```python
from build123d import *

# Parameters (mm, degrees)
F0_R     = 1.671135
F1_DEPTH = 7


with BuildPart() as f1:
    # F0 (on Top) → F1 (new body)
    with BuildSketch(Plane.XY):
        with BuildLine():
            ThreePointArc((5.710763, 3.295388), (5.423242, 3.744527), (5.101476, 4.169805))
            Line((5.101476, 4.169805), (6.17403, 5.210492))
            Line((6.17403, 5.210492), (6.80854, 6.475035))
            ThreePointArc((6.80854, 6.475035), (6.41041, 6.87043), (5.989907, 7.241943))
            Line((5.989907, 7.241943), (4.769408, 6.526365))
            Line((4.769408, 6.526365), (3.800837, 5.388265))
            ThreePointArc((3.800837, 5.388265), (3.355492, 5.681629), (2.888568, 5.939266))
            Line((2.888568, 5.939266), (3.445109, 7.326228))
            Line((3.445109, 7.326228), (3.510427, 8.739523))
            ThreePointArc((3.510427, 8.739523), (2.985895, 8.938801), (2.450639, 9.107161))
            Line((2.450639, 9.107161), (1.626709, 7.957026))
            Line((1.626709, 7.957026), (1.204783, 6.523367))
            ThreePointArc((1.204783, 6.523367), (0.678618, 6.61023), (0.147272, 6.655678))
            Line((0.147272, 6.655678), (0.091568, 8.149096))
            Line((0.091568, 8.149096), (-0.4236, 9.466773))
            ThreePointArc((-0.4236, 9.466773), (-0.983837, 9.435476), (-1.541296, 9.371572))
            Line((-1.541296, 9.371572), (-1.826192, 7.985749))
            Line((-1.826192, 7.985749), (-1.628518, 6.504423))
            ThreePointArc((-1.628518, 6.504423), (-2.144524, 6.369766), (-2.648419, 6.195167))
            Line((-2.648419, 6.195167), (-3.306734, 7.536816))
            Line((-3.306734, 7.536816), (-4.313311, 8.531036))
            ThreePointArc((-4.313311, 8.531036), (-4.812383, 8.274576), (-5.295656, 7.989458))
            Line((-5.295656, 7.989458), (-4.992256, 6.607568))
            Line((-4.992256, 6.607568), (-4.209163, 5.33471))
            ThreePointArc((-4.209163, 5.33471), (-4.625787, 5.001816), (-5.015102, 4.63736))
            Line((-5.015102, 4.63736), (-6.162201, 5.595256))
            Line((-6.162201, 5.595256), (-7.486141, 6.09411))
            ThreePointArc((-7.486141, 6.09411), (-7.837754, 5.656831), (-8.163277, 5.199798))
            Line((-8.163277, 5.199798), (-7.324043, 4.060783))
            Line((-7.324043, 4.060783), (-6.090934, 3.216482))
            ThreePointArc((-6.090934, 3.216482), (-6.336139, 2.742911), (-6.543558, 2.251615))
            Line((-6.543558, 2.251615), (-7.981096, 2.66013))
            Line((-7.981096, 2.66013), (-9.393477, 2.57736))
            ThreePointArc((-9.393477, 2.57736), (-9.536835, 2.034872), (-9.648323, 1.484949))
            Line((-9.648323, 1.484949), (-8.418365, 0.785755))
            Line((-8.418365, 0.785755), (-6.948456, 0.515998))
            ThreePointArc((-6.948456, 0.515998), (-6.979843, -0.016364), (-6.969502, -0.54955))
            Line((-6.969502, -0.54955), (-8.448917, -0.761053))
            Line((-8.448917, -0.761053), (-9.705525, -1.411133))
            ThreePointArc((-9.705525, -1.411133), (-9.615839, -1.96503), (-9.494015, -2.512756))
            Line((-9.494015, -2.512756), (-8.086004, -2.651232))
            Line((-8.086004, -2.651232), (-6.633455, -2.299801))
            ThreePointArc((-6.633455, -2.299801), (-6.445598, -2.798905), (-6.219285, -3.281788))
            Line((-6.219285, -3.281788), (-7.484771, -4.076738))
            Line((-7.484771, -4.076738), (-8.368329, -5.181725))
            ThreePointArc((-8.368329, -5.181725), (-8.061106, -5.651256), (-7.727034, -6.102078))
            Line((-7.727034, -6.102078), (-6.384429, -5.655893))
            Line((-6.384429, -5.655893), (-5.200399, -4.74404))
            ThreePointArc((-5.200399, -4.74404), (-4.82578, -5.123586), (-4.422625, -5.472672))
            Line((-4.422625, -5.472672), (-5.25537, -6.713614))
            Line((-5.25537, -6.713614), (-5.613101, -8.082445))
            ThreePointArc((-5.613101, -8.082445), (-5.141464, -8.386424), (-4.652908, -8.662392))
            Line((-4.652908, -8.662392), (-3.607857, -7.708695))
            Line((-3.607857, -7.708695), (-2.897076, -6.394087))
            ThreePointArc((-2.897076, -6.394087), (-2.400469, -6.588448), (-1.890183, -6.743376))
            Line((-1.890183, -6.743376), (-2.146196, -8.215741))
            Line((-2.146196, -8.215741), (-1.916246, -9.611733))
            ThreePointArc((-1.916246, -9.611733), (-1.361745, -9.6976), (-0.803181, -9.750995))
            Line((-0.803181, -9.750995), (-0.236382, -8.454689))
            Line((-0.236382, -8.454689), (-0.121751, -6.964634))
            ThreePointArc((-0.121751, -6.964634), (0.410976, -6.940203), (0.94016, -6.874185))
            Line((0.94016, -6.874185), (1.305145, -8.323388))
            Line((1.305145, -8.323388), (2.083016, -9.505161))
            ThreePointArc((2.083016, -9.505161), (2.624504, -9.358067), (3.156495, -9.179658))
            Line((3.156495, -9.179658), (3.147036, -7.764886))
            Line((3.147036, -7.764886), (2.645697, -6.357029))
            ThreePointArc((2.645697, -6.357029), (3.12243, -6.11803), (3.579012, -5.842481))
            Line((3.579012, -5.842481), (4.501887, -7.01794))
            Line((4.501887, -7.01794), (5.693177, -7.781155))
            ThreePointArc((5.693177, -7.781155), (6.128022, -7.426536), (6.541455, -7.047171))
            Line((6.541455, -7.047171), (5.957374, -5.758559))
            Line((5.957374, -5.758559), (4.926751, -4.676331))
            ThreePointArc((4.926751, -4.676331), (5.265059, -4.26409), (5.570092, -3.826655))
            Line((5.570092, -3.826655), (6.891282, -4.525123))
            Line((6.891282, -4.525123), (8.290007, -4.737813))
            ThreePointArc((8.290007, -4.737813), (8.543022, -4.236985), (8.766409, -3.722259))
            Line((8.766409, -3.722259), (7.708699, -2.782621))
            Line((7.708699, -2.782621), (6.326996, -2.213148))
            ThreePointArc((6.326996, -2.213148), (6.468383, -1.698945), (6.569123, -1.17526))
            Line((6.569123, -1.17526), (8.060183, -1.275967))
            Line((8.060183, -1.275967), (9.424491, -0.901356))
            ThreePointArc((9.424491, -0.901356), (9.451926, -0.340917), (9.446643, 0.220169))
            Line((9.446643, 0.220169), (8.098191, 0.648361))
            Line((8.098191, 0.648361), (6.604317, 0.606612))
            ThreePointArc((6.604317, 0.606612), (6.524335, 1.133866), (6.403364, 1.653251))
            Line((6.403364, 1.653251), (7.806476, 2.16772))
            Line((7.806476, 2.16772), (8.900465, 3.064858))
            ThreePointArc((8.900465, 3.064858), (8.697577, 3.588004), (8.464537, 4.098432))
            Line((8.464537, 4.098432), (7.058504, 3.941141))
            Line((7.058504, 3.941141), (5.710763, 3.295388))
        make_face()
        Circle(F0_R, mode=Mode.SUBTRACT)
    extrude(amount=F1_DEPTH)


solid = f1.part
```
For this review, take the finished solid that the model builds, in its own axes (mm). A direction names the side the tool comes from. Round coordinates to 2 decimals unless told otherwise and drop trailing zeros.
Q1. Machinability: for faces 1 (the flat face through (-2.973, 6.857, 3.451)), 2 (the flat face through (5.63, 4.68, 3.45)), 3 (the flat face through (-7.065, -5.882, 3.451)), 4 (the cylindrical face through (5.428, 3.738, 3.451)), which of the approach directions +Z, -Z, +X, -X, +Y, -Y give a long, thin tool a straight path to every point of the face, cutting with its end or side? Answer none if there is none.
Findings below:
face 1: +Z, -Z, +Y
face 2: +Z, -Z, +X
face 3: +Z, -Z, -Y
face 4: +Z, -Z
Q2. Insertion check: P1, Ø2, axis at y = 4.5, z = 4, coming from the +X side; P2, Ø1, axis at x = -3, z = 5.5, coming from the -Y side; P3, Ø3, axis at y = 7, z = 4.5, coming from the -X side. Each pin has a flat end and moves straight along its axis. Give the tip position at first contact, or say it passes through.
Findings below:
P1: stops at x = 8.73
P2: stops at y = -7.51
P3: stops at x = -7.95
Q3. Mouldability with a two-part tool opening along Y and no side actions: class faces 5 (the flat face through (-3.803, 8.027, 3.451)), 6 (the cylindrical face through (-9.617, -1.957, 3.451)), 7 (the flat face through (7.028, -2.502, 3.451)) as pulls with the +Y half, pulls with the -Y half, needs draft (parallel to the pull), parting line crosses it, or undercut.
Findings below:
face 5: pulls with the +Y half
face 6: pulls with the -Y half
face 7: undercut
Q4. Wall thickness on line 1 (Y direction, x = -7.75, z = 6); line 2 (Y direction, x = -8.25, z = 3.5); line 3 (X direction, y = 6.75, z = 1.75): over which ranges is each line inside the solid? List them lowest first.
Findings below:
line 1: y = -6.07 to -4.41, -2.57 to -0.66, 0.66 to 2.59, 4.64 to 5.77
line 2: y = -5.37 to -5.03, -2.64 to -0.73, 0.75 to 2.64
line 3: x = -5.02 to -2.92, -1.66 to 0.14, 1.27 to 3.21, 5.15 to 6.54
